Source: CAD feature listing. Evaluate the final solid. Frame: model axes, mm. Give positions to 0.01 mm unless a question says otherwise; leave off trailing zeros. Loops run counter-clockwise (first coordinate to the right, second up) from the corner with the lowest first, then second, coordinate; pieces in that order, holes last. Notation, with made-up numbers: (-3, 0.25) -> (32, 0.25) arc R27 cw to (32, 21.25) -> close; hole circle Ø9 at (-22, 53). An arc over 180 degrees is marked (long way). Answer as a JSON object with one key per item and string values. Group by question number.
from build123d import *

# Parameters (mm, degrees)
F0_W     = 9
F0_H     = 1.5
F1_DEPTH = 10
F3_R     = 1.5
F4_DEPTH = 3
F5_DEPTH = 3.001


with BuildPart() as f1:
    # F0 (on Top) → F1 (new body)
    with BuildSketch(Plane.XY):
        Polygon((4.5, 23.5), (4.5, 22), (15, 22), (15, 25), (-15, 25), (-15, 22), (-4.5, 22), (-4.5, 23.5), align=None)
        with Locations((0, 22.75)):
            Rectangle(F0_W, F0_H)
    extrude(amount=F1_DEPTH)

    # F3 (on offset) → F4 (cut, through all)
    with BuildSketch(Plane(origin=(0, 25, 0), x_dir=(-1, 0, 0), z_dir=(0, 1, 0))):
        with Locations((10.25, 5)):
            Circle(F3_R)
        with Locations((-10.25, 5)):
            Circle(F3_R)
    extrude(amount=-F4_DEPTH, mode=Mode.SUBTRACT)

    # F3 (on offset) → F5 (cut, through all)
    with BuildSketch(Plane(origin=(0, 25, 0), x_dir=(-1, 0, 0), z_dir=(0, 1, 0))):
        with Locations((-22.25, 5)):
            Circle(F3_R)
    extrude(amount=-F5_DEPTH, mode=Mode.SUBTRACT)


solid = f1.part
(1) Material intervals for line 1 (Z direction, x = -10.25, y = 24.2); line 2 (X direction, y = 23.3, z = 4.25), sorted ascending. Write a range as from..to.
(2) First-contact query: pin 1 (5 mm diameter, centred on x = 10.25, z = 5, fed in from -Y). Flat tip, straight axial feed; report the tip coordinate or a pass-through.
(3) Section query C-C on y = 24.4. Return the cut outline in (x, z).
(4) Section query B-B on x = 10.25. Return the cut outline in (y, z), plus the area to 3 significant figures.
(5) Mould query, pull axis Z, two halves, no side actions, for faces 1 (the face through (0, 24, 0)), 2 (the face through (-8.75, 23.52, 5.07)), 3 (the face through (11.75, 23.52, 5.07)), 4 (the face through (0, 24, 10)). Classes: pulls with the +Z half, pulls with the -Z half, needs draft (parallel to the pull), parting line crosses it, or undercut.
(6) Section query A-A on z = 5. Return the cut outline in (x, y), plus the area to 3 significant figures.
Result:
{
 "1": {"line 1": "0..3.5, 6.5..10", "line 2": "-15..-11.55, -8.95..8.95, 11.55..15"},
 "2": {"pin 1": "y = 22"},
 "3": {"outline": "(-15, 0) -> (15, 0) -> (15, 10) -> (-15, 10) -> close; hole circle Ø3 at (-10.25, 5); hole circle Ø3 at (10.25, 5)"},
 "4": {"outline": "(22, 0) -> (25, 0) -> (25, 3.5) -> (22, 3.5) -> close; (22, 6.5) -> (25, 6.5) -> (25, 10) -> (22, 10) -> close", "area": "21.0 mm²"},
 "5": {"face 1": "pulls with the -Z half", "face 2": "undercut", "face 3": "undercut", "face 4": "pulls with the +Z half"},
 "6": {"outline": "(-15, 22) -> (-11.75, 22) -> (-11.75, 25) -> (-15, 25) -> close; (-8.75, 22) -> (8.75, 22) -> (8.75, 25) -> (-8.75, 25) -> close; (11.75, 22) -> (15, 22) -> (15, 25) -> (11.75, 25) -> close", "area": "72.0 mm²"}
}
